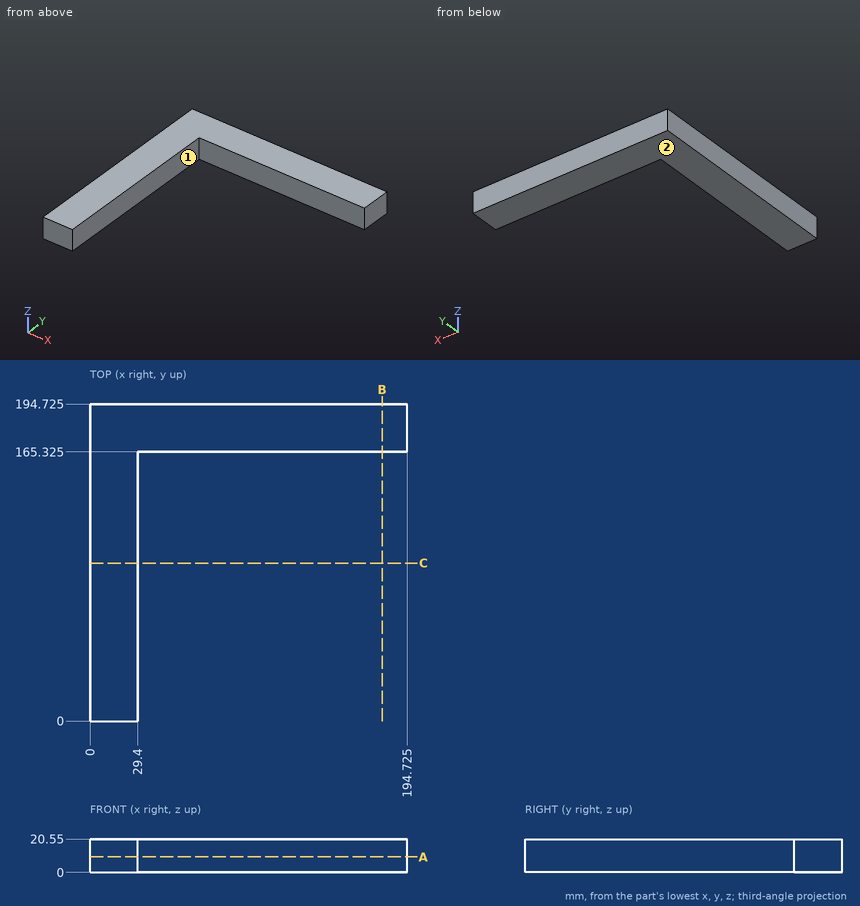
Geometry check sheet. Reference: drawing and pictorial views, mm from the part's lowest x, y, z. A direction names the side the tool comes from. Give positions to 0.01 mm unless a question says otherwise; leave off trailing zeros. Write each loop counter-clockwise with the first axis right and the second up, starting at its lowest first coordinate (ties: lowest second). Pieces come first, ordered by that corner, then holes. Notation, with made-up numbers: (35.25, 13) -> (87.25, 13) arc R30 ccw to (87.25, 46) -> close; hole circle Ø11 at (-16.5, -11.75). An arc over 180 degrees is marked (long way). One line per item, written item: value. Start each with the question number.
Item 1: Tool access check on the marked faces 1 and 2. Record the directions out of +Z, -Z, +X, -X, +Y, -Y that give a thin tool (end or side, any length) a straight path to the whole face; none if there is none.
Item 2: Section check C-C on y = 97. Record the cut outline in (x, z), then the cut area to 3 significant figures.
Item 3: Section check A-A on z = 9.5. Record the cut outline in (x, y) (3 decimals).
Item 4: Section check B-B on x = 179.5. Record the cut outline in (y, z) (3 decimals), then the cut area to 3 significant figures.
Item 5: Gauge pin test, flat end, axial feed: pin 1 (6 mm diameter, centred on x = 146.5, z = 12, fed in from -Y) (3 decimals). Record the tip position at first contact, or that the pin passes through.
Item 6: Material ranges on probe 1 along X at (y, z) = (31, 1.5); probe 2 along Y at (x, z) = (91.5, 7.5) (3 decimals), recorded low to high. Write a range as from..to.
Results list:
1. face 1: +Z, -Z, +X, -Y
1. face 2: -Z, +X, -X, +Y, -Y
2. outline: (0, 0) -> (29.4, 0) -> (29.4, 20.55) -> (0, 20.55) -> close
2. area: 604 mm²
3. outline: (0, 0) -> (29.4, 0) -> (29.4, 165.325) -> (194.725, 165.325) -> (194.725, 194.725) -> (0, 194.725) -> close
4. outline: (165.325, 0) -> (194.725, 0) -> (194.725, 20.55) -> (165.325, 20.55) -> close
4. area: 604 mm²
5. pin 1: y = 165.325
6. probe 1: 0..29.4
6. probe 2: 165.325..194.725
